Part model, mm, in its own coordinate system. A direction names the side the tool comes from. Give positions to 0.01 mm unless a question says otherwise; leave off trailing zeros. Write each loop counter-clockwise with the first axis right and the second up, starting at its lowest first coordinate (ties: lowest second). Pieces come first, ordered by that corner, then holes. Notation, with made-up numbers: M 11,17 L 23,17 A17 cw 23,38 Z; hole C -15.5,22 d6. An arc over 180 degrees is marked long. Use CSV: the item, a comma, the result in double quotes. Start each with the question number.
Item 1: Mould opens along Y. For faces 1 (the flat face through (0, -0.5, 7)), 2 (the flat face through (25.5, -8, 7)), 3 (the flat face through (0, -8.5, 22)), 4 (the flat face through (0, 12, 15)) say: released by +Y, released by -Y, zero draft, split by the parting line, or undercut.
Item 2: Cut at C-C (x = 10). List the corners of the cut face in (y, z).
Item 3: Cut at B-B (z = 16.75). List the corners of the cut face in (x, y), then the cut area to 3 significant figures.
Item 4: Drill centre lines: line 1 (Y direction, x = 3, z = 6); line 2 (X direction, y = -11, z = 12); line 3 (Y direction, x = 11.5, z = 22.5). Where is each one in solid material? Low to high. Write a range as [from, to].
Item 5: Cut at A-A (z = 4). List the corners of the cut face in (x, y), then the cut area to 3 significant figures.
Item 6: Which spindle directions (+Z, -Z, +X, -X, +Y, -Y) get a long thin tool onto all of the face, cutting with end or side? Do faces 5 (the flat face through (0, -12, 15)), 6 (the flat face through (-25.5, -8, 7)), 7 (the flat face through (-25.5, 0, 22)), 8 (the flat face through (26, 0, 11)). Say none if no direction does.
Item 7: Cut at D-D (y = 5). List the corners of the cut face in (x, z), then the cut area to 3 significant figures.
Item 8: Pin check, flat tips, straight feed: pin 1 (4 mm diameter, centred on x = -1, y = -5.5, fed in from -Z); pin 2 (11 mm diameter, centred on x = -2, z = 23, fed in from +Y); pin 3 (2 mm diameter, centred on x = -11.5, y = 3, fed in from +Z). Stop position of each tip, or through.
Autodesk Inventor part; units mm, degrees
ref_plane "YZ Plane" through (0, 0, 0) normal (1, 0, 0) x (0, 1, 0)
ref_plane "XZ Plane" through (0, 0, 0) normal (0, 1, 0) x (-1, 0, 0)
ref_plane "XY Plane" through (0, 0, 0) normal (0, 0, 1) x (1, 0, 0)
sketch "Szkic1" plane through (0, 0, 0) normal (0, 0, 1) x (1, 0, 0)
  line L0 (25.5, -15.5) -> (-25.5, -15.5)
  line L1 (-25.5, -15.5) -> (-25.5, 15.5)
  line L2 (-25.5, 15.5) -> (25.5, 15.5)
  line L3 (25.5, 15.5) -> (25.5, -15.5)
  line L4 (25.5, -15.5) -> (-25.5, 15.5) construction
  line L5 (-25.5, -15.5) -> (25.5, 15.5) construction
  line L6 (26, -16) -> (-26, -16)
  line L7 (-26, -16) -> (-26, 16)
  line L8 (-26, 16) -> (26, 16)
  line L9 (26, 16) -> (26, -16)
  line L10 (26, -16) -> (-26, 16) construction
  line L11 (-26, -16) -> (26, 16) construction
  point P0 (0, 0)
  dimension "d0" = 51
  dimension "d1" = 31
  dimension "d2" = 52
  dimension "d3" = 32
extrude "Wyciągnięcie proste1" add sketch "Szkic1" along normal blind 15
sketch "Szkic2" plane through (0, 0, 15) normal (0, 0, 1) x (1, 0, 0)
  line L0 (-25.5, -15.5) -> (-25.5, 15.5)
  line L1 (25.5, -15.5) -> (-25.5, -15.5)
  line L2 (-25.5, -15.5) -> (-25.5, 15.5)
  line L3 (-25.5, 15.5) -> (25.5, 15.5)
  line L4 (25.5, 15.5) -> (25.5, -15.5)
  line L5 (25.5, -15.5) -> (-25.5, 15.5) construction
  line L6 (-25.5, -15.5) -> (25.5, 15.5) construction
  point P0 (0, 0)
extrude "Wyciągnięcie proste2" add sketch "Szkic2" against normal blind 1
sketch "Szkic4" plane through (0, 0, 14) normal (0, 0, -1) x (-1, 0, 0)
  line L0 (-25.5, -15.5) -> (-25.5, 15.5)
  line L1 (-25.5, 0) -> (-25.5, 0.5)
  line L2 (-25.5, 0.5) -> (25.5, 0.5)
  line L3 (25.5, 15.5) -> (25.5, -15.5)
  line L4 (25.5, -0.5) -> (-25.5, -0.5)
  point P0 (0, 0)
  dimension "d14" = 0.5
extrude "Wyciągnięcie proste4" add sketch "Szkic4" along normal blind 14
sketch "Szkic5" plane through (0, 0, 15) normal (0, 0, 1) x (1, 0, 0)
  line L0 (0, 0) -> (0, 7.5)
  line L1 (0, 7.5) -> (0, 8.5)
  line L2 (0, 8.5) -> (26, 8.5)
  line L3 (26, -16) -> (26, 16)
  line L4 (0, 8.5) -> (-26, 8.5)
  line L5 (-26, 16) -> (-26, -16)
  line L6 (25.5, -0.5) -> (-25.5, -0.5)
  line L7 (0, 0) -> (0, -7.5)
  line L8 (0, -7.5) -> (26, -7.5)
  line L9 (0, -7.5) -> (-26, -7.5)
  line L10 (0, 7.5) -> (26, 7.5)
  line L11 (26, 8.5) -> (26, 7.5)
  line L12 (0, 7.5) -> (-26, 7.5)
  line L13 (-26, 8.5) -> (-26, 7.5)
  line L14 (-26, -7.5) -> (-26, -8.5)
  line L15 (-26, -8.5) -> (26, -8.5)
  line L16 (26, -7.5) -> (26, -8.5)
  line L17 (26, -7.5) -> (26, 7.5)
  line L18 (-26, 7.5) -> (-26, -7.5)
  dimension "d17" = 7.5
  dimension "d18" = 1
  dimension "d20" = 7.5
  dimension "d21" = 1
extrude "Wyciągnięcie proste5" add sketch "Szkic5" along normal blind 14 contours L12 L5 L4 L1 | L1 L2 L3 L10 | L8 L3 L15 L5 L9
sketch "Szkic7" plane through (0, 0, 15) normal (0, 0, 1) x (1, 0, 0)
  line L0 (26, 7.5) -> (-26, 7.5)
  line L1 (-26, 7.5) -> (-25.5, 7.5)
  line L2 (-25.5, 7.5) -> (-25.5, -7.5)
  line L3 (-25.5, -15.5) -> (-25.5, -0.5)
  line L4 (26, -7.5) -> (-26, -7.5)
  line L5 (-25.5, -7.5) -> (-26, -7.5)
  line L6 (-26, 8.5) -> (-26, 7.5)
  line L7 (-26, -7.5) -> (-26, 7.5)
  line L8 (26, 7.5) -> (25.5, 7.5)
  line L9 (25.5, 15.5) -> (25.5, 0.5)
  line L10 (25.5, 7.5) -> (25.5, -7.5)
  line L11 (25.5, -0.5) -> (25.5, -15.5)
  line L12 (25.5, -7.5) -> (26, -7.5)
  line L13 (26, -7.5) -> (26, 7.5)
  line L14 (26, -16) -> (26, 16)
  point P0 (0, 0)
  point P1 (25.5, 0.5)
  dimension "d30" = 0.5
  dimension "d31" = 15
extrude "Wyciągnięcie proste7" add sketch "Szkic7" along normal blind 14 contours L13 L4 L10 L9 L0 | L2 L4 L7 L0
properties part number "Magazynek na baterie"
Worked answers:
1,face 1,"undercut"
1,face 2,"undercut"
1,face 3,"released by -Y"
1,face 4,"zero draft"
2,outline,"M -16,0 L -15.5,0 L -15.5,14 L -0.5,14 L -0.5,0 L 0.5,0 L 0.5,14 L 15.5,14 L 15.5,0 L 16,0 L 16,15 L 8.5,15 L 8.5,29 L 7.5,29 L 7.5,15 L -7.5,15 L -7.5,29 L -8.5,29 L -8.5,15 L -16,15 Z"
3,outline,"M -26,-8.5 L 26,-8.5 L 26,8.5 L -26,8.5 Z; hole M -25.5,-7.5 L 25.5,-7.5 L 25.5,7.5 L -25.5,7.5 Z"
3,area,"119 mm^2"
4,line 1,"y = [-16, -15.5], [-0.5, 0.5], [15.5, 16]"
4,line 2,"x = [-26, -25.5], [25.5, 26]"
4,line 3,"y = [-8.5, -7.5], [7.5, 8.5]"
5,outline,"M -26,-16 L 26,-16 L 26,16 L -26,16 Z; hole M -25.5,-15.5 L 25.5,-15.5 L 25.5,-0.5 L -25.5,-0.5 Z; hole M -25.5,0.5 L 25.5,0.5 L 25.5,15.5 L -25.5,15.5 Z"
5,area,"134 mm^2"
6,face 5,"+Z, +X, -X, -Y"
6,face 6,"-Z"
6,face 7,"+Z"
6,face 8,"+Z, -Z, +X, +Y, -Y"
7,outline,"M -26,0 L -25.5,0 L -25.5,14 L 25.5,14 L 25.5,0 L 26,0 L 26,29 L 25.5,29 L 25.5,15 L -25.5,15 L -25.5,29 L -26,29 Z"
7,area,"80.0 mm^2"
8,pin 1,"stops at z = 14"
8,pin 2,"stops at y = 8.5"
8,pin 3,"stops at z = 15"
